CAD build for the part. Positions are in the model's coordinates, mm. Face numbers are marked on the shaded views. A direction names the side the tool comes from. Give positions to 0.01 mm unless a question says otherwise; leave off trailing zeros. Loops run counter-clockwise (first coordinate to the right, second up) from the corner with the lowest first, then second, coordinate; pieces in that order, holes last. Notation, with made-up numbers: (-38, -1.5) -> (20, -1.5) arc R18 ccw to (20, 4.5) -> close; hole circle Ø9 at (89, 85.5). An arc over 180 degrees is marked (long way). Use one line per item in the form item = value.
```python
from build123d import *

# Parameters (mm, degrees)
SKETCH1_W                = 11
SKETCH1_H                = 25
BOSS_EXTRUDE1_DEPTH      = 35
CUT_EXTRUDE9_DEPTH       = 31.868357473
CUT_EXTRUDE9_DEPTH_BACK  = 31.868357473
SKETCH6_R                = 20
SKETCH6_R_2              = 12.5
SKETCH7_W                = 11
SKETCH7_H                = 20
BOSS_EXTRUDE3_DEPTH      = 20
SKETCH8_R                = 15
SKETCH8_R_2              = 10
CUT_EXTRUDE10_DEPTH      = 51.682837382
CUT_EXTRUDE11_DEPTH      = 40.210967919
CUT_EXTRUDE11_DEPTH_BACK = 40.210967919
SKETCH9_W                = 4
SKETCH9_H                = 20
SKETCH9_H_2              = 22.5
CUT_EXTRUDE15_START      = -3.5
CUT_EXTRUDE15_DEPTH      = 11
CUT_EXTRUDE16_DEPTH      = 40.893608668
CUT_EXTRUDE16_DEPTH_BACK = 40.893608668
CUT_EXTRUDE17_DEPTH      = 42.29467294
CUT_EXTRUDE17_DEPTH_BACK = 42.29467294
SKETCH14_R               = 3
SKETCH15_W               = 6
SKETCH15_H               = 8
BOSS_EXTRUDE5_DEPTH      = 18
SKETCH17_R               = 2
CUT_EXTRUDE19_DEPTH      = 45.735332948
SKETCH20_W               = 6
SKETCH20_H               = 6
BOSS_EXTRUDE7_DEPTH      = 18
SKETCH21_R               = 2
CUT_EXTRUDE22_DEPTH      = 50.603427453
SCALE1_SCALE             = 0.75


# Read off the part's stored shape, not the designer's step: Cut-Extrude15
with BuildPart() as part:
    # Sketch1 → Boss-Extrude1 (new body)
    with BuildSketch(Plane.XY):
        Rectangle(SKETCH1_W, SKETCH1_H)
    extrude(amount=BOSS_EXTRUDE1_DEPTH)


with BuildPart() as body_2:
    # Sketch2 → Revolve1 (revolve)
    with BuildSketch(Plane(origin=(0, 0, 0), x_dir=(0, 0, -1), z_dir=(1, 0, 0))):
        with BuildLine():
            Line((-12.5, 0), (12.5, 0))
            Line((12.5, 0), (12.5, 10))
            add(Edge.make_bspline(
                [(-12.5, 12.5), (0.245145169, 13.725725845), (12.5, 10)],
                knots=[0, 0, 0, 1, 1, 1], degree=2))
            Line((-12.5, 12.5), (-12.5, 0))
        make_face()
    revolve(axis=Axis((0, 0, 12.5), (0, 0, -1)))


with BuildPart() as cut_extrude9_tool:
    # Sketch6 → Cut-Extrude9 (new, two sides: drawn at the far end of the back side and taken through both)
    with BuildSketch(Plane.XY.offset(12.5).offset(-CUT_EXTRUDE9_DEPTH_BACK)):
        Circle(SKETCH6_R)
        with Locations(Location((0, 0, 0), (0, 0, 270))):
            Circle(SKETCH6_R_2, mode=Mode.SUBTRACT)
    extrude(amount=CUT_EXTRUDE9_DEPTH + CUT_EXTRUDE9_DEPTH_BACK)


with BuildPart() as part_1:
    add(part.part)

    # Cut-Extrude9: cut by cut_extrude9_tool
    add(cut_extrude9_tool.part, mode=Mode.SUBTRACT)


with BuildPart() as body_2_1:
    add(body_2.part)

    # Cut-Extrude9: cut by cut_extrude9_tool
    add(cut_extrude9_tool.part, mode=Mode.SUBTRACT)

    # Sketch7 → Boss-Extrude3 (add)
    with BuildSketch(Plane(origin=(0, 0, -12.5), x_dir=(-1, 0, 0), z_dir=(0, 0, -1))):
        Rectangle(SKETCH7_W, SKETCH7_H)
    extrude(amount=BOSS_EXTRUDE3_DEPTH)

    # Sketch8 → Cut-Extrude10 (cut, through all)
    with BuildSketch(Plane(origin=(0, 0, -12.5), x_dir=(-1, 0, 0), z_dir=(0, 0, -1))):
        Circle(SKETCH8_R)
        Circle(SKETCH8_R_2, mode=Mode.SUBTRACT)
    extrude(amount=CUT_EXTRUDE10_DEPTH, mode=Mode.SUBTRACT)


with BuildPart() as cut_extrude11_tool:
    # Sketch9 → Cut-Extrude11 (new, two sides: drawn at the far end of the back side and taken through both)
    with BuildSketch(Plane(origin=(0, 0, 0), x_dir=(1, 0, 0), z_dir=(0, 1, 0)).offset(-CUT_EXTRUDE11_DEPTH_BACK)):
        with Locations((0, 22.5)):
            Rectangle(SKETCH9_W, SKETCH9_H)
        with Locations((0, -23.75)):
            Rectangle(SKETCH9_W, SKETCH9_H_2)
    extrude(amount=CUT_EXTRUDE11_DEPTH + CUT_EXTRUDE11_DEPTH_BACK)


with BuildPart() as part_2:
    add(part_1.part)

    # Cut-Extrude11: cut by cut_extrude11_tool
    add(cut_extrude11_tool.part, mode=Mode.SUBTRACT)

    # Cut-Extrude15 outline → Cut-Extrude15 (cut)
    with BuildSketch(Plane(origin=(-2, 0, 0), x_dir=(0, 0, -1), z_dir=(1, 0, 0)).offset(CUT_EXTRUDE15_START)):
        with BuildLine():
            Line((-35, 12.338962679), (-35, -1.7e-08))
            ThreePointArc((-35, -1.7e-08), (-31.38600151, 8.724964177), (-22.661037321, 12.338962679))
            Line((-22.661037321, 12.338962679), (-35, 12.338962679))
        make_face()
        with BuildLine():
            Line((-35, -12.338962679), (-22.661037321, -12.338962679))
            ThreePointArc((-22.661037321, -12.338962679), (-31.386001498, -8.724964189), (-35, -1.7e-08))
            Line((-35, -1.7e-08), (-35, -12.338962679))
        make_face()
    extrude(amount=CUT_EXTRUDE15_DEPTH, mode=Mode.SUBTRACT)


with BuildPart() as body_2_2:
    add(body_2_1.part)

    # Cut-Extrude11: cut by cut_extrude11_tool
    add(cut_extrude11_tool.part, mode=Mode.SUBTRACT)

    # Sketch12 → Cut-Extrude16 (cut, two sides: drawn at the far end of the back side and taken through both)
    with BuildSketch(Plane.ZY.offset(-2).offset(-CUT_EXTRUDE16_DEPTH_BACK)):
        with BuildLine():
            ThreePointArc((-32.5, 0), (-29.630244259, 6.92820323), (-22.702041029, 9.797958971))
            Line((-22.702041029, 9.797958971), (-32.5, 9.797958971))
            Line((-32.5, 9.797958971), (-32.5, 0))
        make_face()
        with BuildLine():
            ThreePointArc((-22.702041029, -9.797958971), (-29.630244259, -6.92820323), (-32.5, 0))
            Line((-32.5, 0), (-32.5, -9.797958971))
            Line((-32.5, -9.797958971), (-22.702041029, -9.797958971))
        make_face()
    extrude(amount=CUT_EXTRUDE16_DEPTH + CUT_EXTRUDE16_DEPTH_BACK, mode=Mode.SUBTRACT)


with BuildPart() as cut_extrude17_tool:
    # Sketch14 → Cut-Extrude17 (new, two sides: drawn at the far end of the back side and taken through both)
    with BuildSketch(Plane.ZY.offset(5.5).offset(-CUT_EXTRUDE17_DEPTH_BACK)):
        with Locations(Location((-22.702041029, 0, 0), (0, 0, 270))):
            Circle(SKETCH14_R)
        with Locations(Location((25.202041029, 0, 0), (0, 0, 270))):
            Circle(SKETCH14_R)
    extrude(amount=CUT_EXTRUDE17_DEPTH + CUT_EXTRUDE17_DEPTH_BACK)


with BuildPart() as part_3:
    add(part_2.part)

    # Cut-Extrude17: cut by cut_extrude17_tool
    add(cut_extrude17_tool.part, mode=Mode.SUBTRACT)



with BuildPart() as body_2_3:
    add(body_2_2.part)

    # Cut-Extrude17: cut by cut_extrude17_tool
    add(cut_extrude17_tool.part, mode=Mode.SUBTRACT)


with BuildPart() as part_4:
    add(part_3.part)

    add(body_2_3.part)  # Boss-Extrude5 merges body 2
    # Sketch15 → Boss-Extrude5 (add)
    with BuildSketch(Plane(origin=(0, 0, 0), x_dir=(1, 0, 0), z_dir=(0, 1, 0))):
        Rectangle(SKETCH15_W, SKETCH15_H)
    extrude(amount=-BOSS_EXTRUDE5_DEPTH)

    # Sketch17 → Cut-Extrude19 (cut, through all)
    with BuildSketch(Plane(origin=(0, 0, -4), x_dir=(-1, 0, 0), z_dir=(0, 0, -1))):
        with Locations((0, -14.989547851)):
            Circle(SKETCH17_R)
    extrude(amount=-CUT_EXTRUDE19_DEPTH, mode=Mode.SUBTRACT)

    # Sketch20 → Boss-Extrude7 (add)
    with BuildSketch(Plane(origin=(0, 0, 0), x_dir=(1, 0, 0), z_dir=(0, 1, 0))):
        with Locations((0, 9)):
            Rectangle(SKETCH20_W, SKETCH20_H)
        with Locations((0, -9)):
            Rectangle(SKETCH20_W, SKETCH20_H)
    extrude(amount=BOSS_EXTRUDE7_DEPTH)

    # Sketch21 → Cut-Extrude22 (cut, through all)
    with BuildSketch(Plane.XY.offset(12)):
        with Locations((0, 15.25)):
            Circle(SKETCH21_R)
    extrude(amount=-CUT_EXTRUDE22_DEPTH, mode=Mode.SUBTRACT)


with BuildPart() as part_5:
    # Scale1: scaled about (2.31e-07, 0.10771387, 1.886694497)
    add(part_4.part.scale(SCALE1_SCALE).moved(Location((5.8e-08, 0.026928468, 0.471673624))))


solid = part_5.part
```
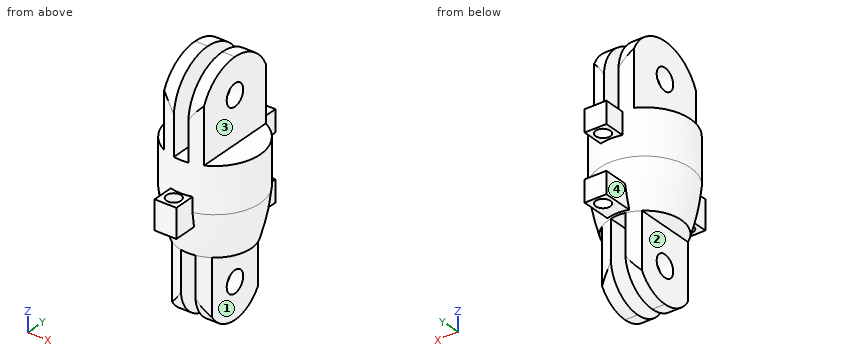
1. Cut at D-D, the plane x = 0. State how many separate pieces and enclosed holes the cut face has, then the cut area to 3 significant figures.
Result sheet:
separate_pieces = 4
enclosed_holes = 0
area = 360 mm^2
2. Drop flat-ended pins along their axis: P1, Ø2, axis at y = -3, z = 5.5, coming from the -X side; P2, Ø10, axis at y = -8.5, z = -13.5, coming from the -X side (3 decimals); P3, Ø10, axis at x = -5.5, y = 9.5, coming from the -Z side. Give the stop position or say it passes through.
Result sheet:
P1 = -9.15
P2 = -4.125
P3 = -22.23
3. Drill centre lines: line 1 (Z direction, x = 0, y = 9.5); line 2 (X direction, y = 6.75, z = 12) (3 decimals); line 3 (Z direction, x = 1.5, y = -10). Where is each one in solid material? Low to high.
Result sheet:
line_1 = -8.53 to -4.03, 4.97 to 9.47
line_2 = -4.125 to -1.5, 1.5 to 4.125
line_3 = -2.53 to 3.47
4. Cut at B-B, the plane z = -18. Write the cut outline in (x, y) (3 decimals), then the cut area to 3 significant figures.
Result sheet:
outline = (-4.125, -6.237) arc R7.5 ccw to (-2.083, -7.178) -> (-1.5, -7.178) -> (-1.5, -1.698) -> (-4.125, -1.698) -> close; (-4.125, 1.751) -> (-1.5, 1.751) -> (-1.5, 7.232) -> (-2.083, 7.232) arc R7.5 ccw to (-4.125, 6.291) -> close; (1.5, -7.178) -> (2.083, -7.178) arc R7.5 ccw to (4.125, -6.237) -> (4.125, -1.698) -> (1.5, -1.698) -> close; (1.5, 1.751) -> (4.125, 1.751) -> (4.125, 6.291) arc R7.5 ccw to (2.083, 7.232) -> (1.5, 7.232) -> close
area = 54.2 mm^2
5. Cut at C-C, the plane z = 8.5. Write the cut outline in (x, y) (3 decimals), then the cut area to 3 significant figures.
Result sheet:
outline = (-2.25, 9.128) arc R9.375 ccw (long way) to (2.25, 9.128) -> (2.25, 13.527) -> (-2.25, 13.527) -> close; hole circle Ø3 at (0, 11.464)
area = 288 mm^2
6. Cut at A-A, the plane z = 14.5. Write the cut outline in (x, y) (3 decimals), then the cut area to 3 significant figures.
Result sheet:
outline = (-4.125, -8.392) arc R9.375 ccw to (-1.5, -9.227) -> (-1.5, 9.281) arc R9.375 ccw to (-4.125, 8.446) -> close; (1.5, -9.227) arc R9.375 ccw to (4.125, -8.392) -> (4.125, 8.446) arc R9.375 ccw to (1.5, 9.281) -> close
area = 93.5 mm^2
7. Tool access for the marked faces 1, 2, 3 and 4: list every direction of +Z, -Z, +X, -X, +Y, -Y with a clear straight run to the whole face (end or side of a thin tool).
Result sheet:
face_1 = -Z, +X, +Y, -Y
face_2 = -Z, -X, +Y, -Y
face_3 = +Z, +X, +Y, -Y
face_4 = -Z, -X, +Y
